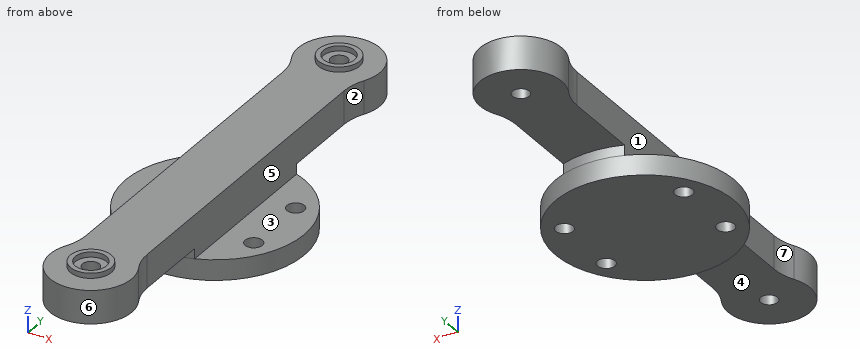
```python
from build123d import *

# Parameters (mm, degrees)
SKETCH_1_W                   = 17.5
SKETCH_1_H                   = 4
EXTRUDE_1_DEPTH              = 2
EXTRUDE_2_DEPTH              = 6.5
SKETCH_4_W                   = 4
SKETCH_4_H                   = 1
SKETCH_5_W                   = 4
SKETCH_5_H                   = 1
HOLE_WIZARD_3_4_3_4_1_D      = 3.4
HOLE_WIZARD_3_4_3_4_1_DEPTH  = 13.5
HOLE_WIZARD_M3_1_D           = 3.3
HOLE_WIZARD_M3_1_DEPTH       = 13.5
HOLE_WIZARD_M3_1_CBORE_D     = 6.1
HOLE_WIZARD_M3_1_CBORE_DEPTH = 1
FILLET_1_R                   = 10


with BuildPart() as part:
    # 草图1 → 旋转1 (revolve)
    with BuildSketch(Plane(origin=(0, 0, 0), x_dir=(1, 0, 0), z_dir=(0, 1, 0))):
        with Locations((8.75, 2)):
            Rectangle(SKETCH_1_W, SKETCH_1_H)
    revolve(axis=Axis((0, 0, -4), (0, 0, 1)))

    # 草图2 → 凸台-拉伸1 (add)
    with BuildSketch(Plane.XY):
        with BuildLine():
            Line((6, 16.439282223), (6, -16.439282223))
            ThreePointArc((6, -16.439282223), (0, -17.5), (-6, -16.439282223))
            Line((-6, -16.439282223), (-6, 16.439282223))
            ThreePointArc((-6, 16.439282223), (0, 17.5), (6, 16.439282223))
        make_face()
    extrude(amount=EXTRUDE_1_DEPTH)

    # 草图3 → 凸台-拉伸2 (add)
    with BuildSketch(Plane.XY.offset(2)):
        with BuildLine():
            Line((-6, -34.708497378), (-6, 34.708497378))
            ThreePointArc((-6, 34.708497378), (0, 48), (6, 34.708497378))
            Line((6, 34.708497378), (6, -34.708497378))
            ThreePointArc((6, -34.708497378), (0, -48), (-6, -34.708497378))
        make_face()
    extrude(amount=EXTRUDE_2_DEPTH)

    # 草图4 → 旋转2 (revolve)
    with BuildSketch(Plane.XZ.offset(40), mode=Mode.PRIVATE) as revolve_2_sk:
        with Locations((2, 9)):
            Rectangle(SKETCH_4_W, SKETCH_4_H)
    revolve(revolve_2_sk.sketch.rotate(Axis((0, -40, 9.5), (0, 0, -1)), 180), axis=Axis((0, -40, 9.5), (0, 0, -1)))

    # 草图5 → 旋转3 (revolve)
    with BuildSketch(Plane.XZ.offset(-40), mode=Mode.PRIVATE) as revolve_3_sk:
        with Locations((2, 9)):
            Rectangle(SKETCH_5_W, SKETCH_5_H)
    revolve(revolve_3_sk.sketch.rotate(Axis((0, 40, 9.5), (0, 0, -1)), 180), axis=Axis((0, 40, 9.5), (0, 0, -1)))

    # Ø3.4 (3.4) 直径孔1
    with Locations(Plane(origin=(0, 0, -4), x_dir=(-1, 0, 0), z_dir=(0, 0, -1))):
        with Locations((11.691342951, 6.75), (11.691342951, -6.75), (-11.691342951, -6.75), (-11.691342951, 6.75)):
            Hole(HOLE_WIZARD_3_4_3_4_1_D / 2, depth=HOLE_WIZARD_3_4_3_4_1_DEPTH)

    # M3 六角头机械螺钉的柱形沉头孔1
    with Locations(Plane.XY.offset(9.5)):
        with Locations((0, -40), (0, 40)):
            CounterBoreHole(HOLE_WIZARD_M3_1_D / 2, HOLE_WIZARD_M3_1_CBORE_D / 2, HOLE_WIZARD_M3_1_CBORE_DEPTH, depth=HOLE_WIZARD_M3_1_DEPTH)

    # 圆角1
    fillet_1_edges = [part.edges().sort_by_distance(p)[0] for p in [
        (-6, -34.708497378, 5.25),
        (6, -34.708497378, 5.25),
        (6, 34.708497378, 5.25),
        (-6, 34.708497378, 5.25),
    ]]
    fillet(fillet_1_edges, radius=FILLET_1_R)


solid = part.part
```
The listing builds one solid part. Answer for the finished solid, in the listing's coordinates (mm). Face numbers are marked on the shaded views. A direction names the side the tool comes from. Round coordinates to 2 decimals unless told otherwise and drop trailing zeros. Loops run counter-clockwise (first coordinate to the right, second up) from the corner with the lowest first, then second, coordinate; pieces in that order, holes last. Notation, with made-up numbers: (-13.5, 88.5) -> (29.5, 88.5) arc R34 cw to (29.5, 121.5) -> close; hole circle Ø8 at (-10.5, 43.5). An arc over 180 degrees is marked (long way). Use one line per item in the form item = value.
1. A tool of negligible diameter and unlimited length cuts with its end or side. For the marked faces 1, 2 and 3, from which of +Z, -Z, +X, -X, +Y, -Y can it reach the whole face along a straight path? Write none if from no direction.
Answer key:
face_1 = +Z, -X
face_2 = +Z, -Z, +X
face_3 = +Z, +X, +Y, -Y
2. The part is cut by section A-A on x = 0. Give the number of separate pieces and of enclosed holes in the cut face, and give its area (3 significant figures).
Answer key:
separate_pieces = 3
enclosed_holes = 0
area = 795 mm²
3. For a pull along X with two mould halves and no side action, classify the marked faces 4, 5, 6 and 7 as released by +X, released by -X, zero draft, split by the parting line, or undercut.
Answer key:
face_4 = zero draft
face_5 = released by +X
face_6 = split by the parting line
face_7 = released by -X
4. The part is cut by section D-D on y = 0. Determine the outline of the cut face in (x, z).
Answer key:
outline = (-17.5, -4) -> (17.5, -4) -> (17.5, 0) -> (6, 0) -> (6, 8.5) -> (-6, 8.5) -> (-6, 0) -> (-17.5, 0) -> close
5. Find the intervals of material crossed by probe 1 along Y at (x, z) = (0, 9.1); probe 2 along Y at (x, z) = (0, 6.5); probe 3 along X at (y, z) = (8, -2.5), in increasing order. Write a range as [from, to].
Answer key:
probe_1 = [-44, -43.05], [-36.95, -36], [36, 36.95], [43.05, 44]
probe_2 = [-48, -41.65], [-38.35, 38.35], [41.65, 48]
probe_3 = [-15.56, -12.84], [-10.54, 10.54], [12.84, 15.56]
6. The part is cut by section B-B on z = 6.75. Determine the outline of the cut face in (x, y), and give its area (3 significant figures).
Answer key:
outline = (-7.11, -36.34) arc R8 ccw (long way) to (7.11, -36.34) arc R10 cw to (6, -31.75) -> (6, 31.75) arc R10 cw to (7.11, 36.34) arc R8 ccw (long way) to (-7.11, 36.34) arc R10 cw to (-6, 31.75) -> (-6, -31.75) arc R10 cw to start; hole circle Ø3.3 at (0, -40); hole circle Ø3.3 at (0, 40)
area = 1,180 mm²
7. The part is cut by section C-C on y = 40. Determine the outline of the cut face in (x, z).
Answer key:
outline = (-8, 2) -> (-1.65, 2) -> (-1.65, 8.5) -> (-3.05, 8.5) -> (-3.05, 9.5) -> (-4, 9.5) -> (-4, 8.5) -> (-8, 8.5) -> close; (1.65, 2) -> (8, 2) -> (8, 8.5) -> (4, 8.5) -> (4, 9.5) -> (3.05, 9.5) -> (3.05, 8.5) -> (1.65, 8.5) -> close
8. Flat-ended cylindrical pins translate along their axes: pin 1 Ø1.8 at (x, y) = (-0.5, -38.5) entering from +Z; pin 2 Ø8 at (x, z) = (5.5, 6) entering from +Y; pin 3 Ø7 at (y, z) = (-8, 4) entering from +X. Find the tip coordinate at first contact, or state that the pin passes through.
Answer key:
pin_1 = 8.5
pin_2 = 47.86
pin_3 = 6
